Print and shaded views of the part. All mm, measured from the part's lowest x, y and z. A direction names the side the tool comes from. Round coordinates to 2 decimals unless told otherwise and drop trailing zeros. Order: outer loops, then holes, each group sorted by start corner. A loop starts at its lowest first (then second) coordinate and runs counter-clockwise, first axis right, second up. Notation, with made-up numbers: (-25, 27) - (-21, 27) arc R11 cw to (-21, 41) - close; hole circle Ø1 at (19, 23). An arc over 180 degrees is marked (long way). Return JSON: item names as keys, results as strings. Group by question number.
Item 1: Saw through at B-B on z = 11.5. List the corners of the cut face in (x, y) (3 decimals), and give its area (3 significant figures).
Item 2: Drop flat-ended pins along their axis: pin 1 (12.5 mm diameter, centred on x = 647.065, z = 32.385, fed in from +Y); pin 2 (22.5 mm diameter, centred on x = 412.75, z = 32.385, fed in from +Y); pin 3 (6 mm diameter, centred on y = 197.5, z = 36.5, fed in from -X). Give the stop position or say it passes through.
Item 3: Tool access for the marked faces 1 and 2: list every direction of +Z, -Z, +X, -X, +Y, -Y with a clear straight run to the whole face (end or side of a thin tool).
Item 4: Probe probe 1 along Y at (x, z) = (658.5, 27) (3 decimals); probe 2 along Z at (x, y) = (412.75, 6.75); probe 3 along X at (y, z) = (75.5, 79.5). List the from-to ranges inside material, lowest first.
Item 5: Two-plate mould, pull along X, no slides. Class the marked faces 3, 4, 5 and 6: released by +X, released by -X, zero draft, split by the parting line, or undercut.
Item 6: Saw through at A-A on y = 661. List the corners of the cut face in (x, z), and give its area (3 significant figures).
Item 7: Saw through at C-C on y = 357. List the corners of the cut face in (x, z).
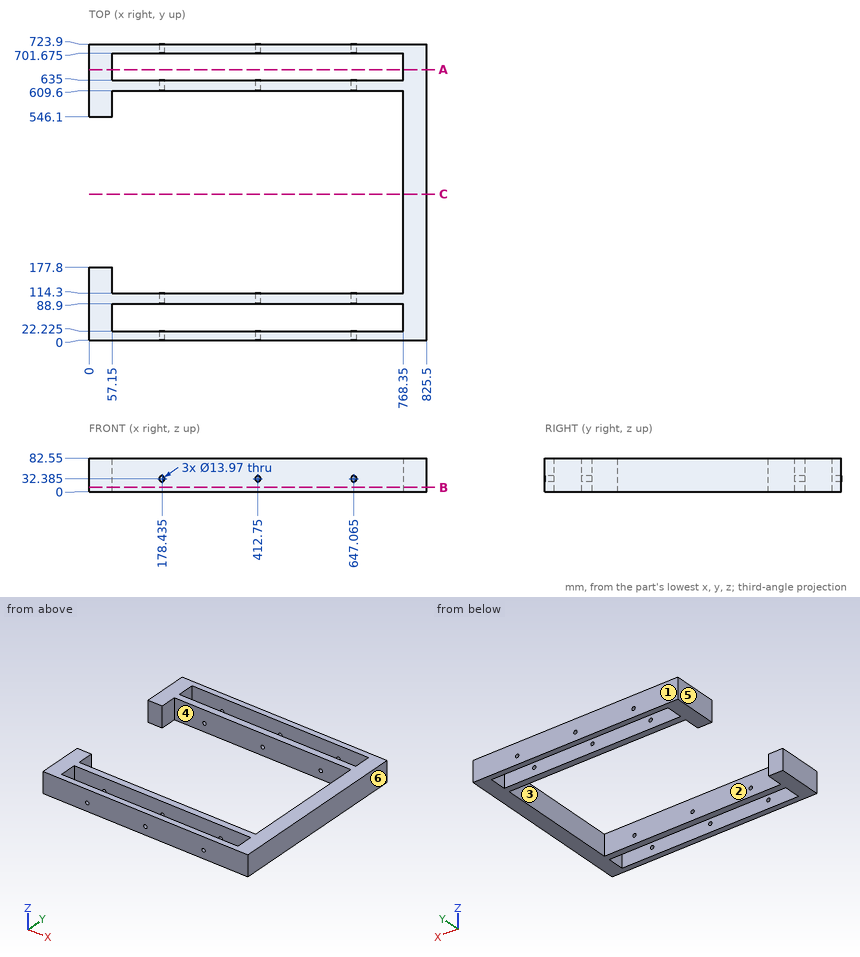
Filled in:
{
 "1": {"outline": "(0, 0) - (825.5, 0) - (825.5, 723.9) - (0, 723.9) - (0, 546.1) - (57.15, 546.1) - (57.15, 609.6) - (768.35, 609.6) - (768.35, 114.3) - (57.15, 114.3) - (57.15, 177.8) - (0, 177.8) - close; hole (57.15, 22.225) - (768.35, 22.225) - (768.35, 88.9) - (57.15, 88.9) - close; hole (57.15, 635) - (768.35, 635) - (768.35, 701.675) - (57.15, 701.675) - close", "area": "129,000 mm^2"},
 "2": {"pin 1": "passes through", "pin 2": "stops at y = 723.9", "pin 3": "stops at x = 768.35"},
 "3": {"face 1": "+Z, -Z, +X, -X, +Y", "face 2": "+Z, -Z"},
 "4": {"probe 1": "y = 0 to 22.225, 88.9 to 114.3, 609.6 to 635, 701.675 to 723.9", "probe 2": "z = 0 to 25.4, 39.37 to 82.55", "probe 3": "x = 0 to 57.15, 768.35 to 825.5"},
 "5": {"face 3": "undercut", "face 4": "undercut", "face 5": "released by -X", "face 6": "released by +X"},
 "6": {"outline": "(0, 0) - (57.15, 0) - (57.15, 82.55) - (0, 82.55) - close; (768.35, 0) - (825.5, 0) - (825.5, 82.55) - (768.35, 82.55) - close", "area": "9,440 mm^2"},
 "7": {"outline": "(768.35, 0) - (825.5, 0) - (825.5, 82.55) - (768.35, 82.55) - close"}
}
